from build123d import *

# Parameters (mm, degrees)
F0_W     = 50
F0_H     = 100
F1_DEPTH = 1000
F2_R     = 5.5
F3_T     = -2.5


with BuildPart() as f1:
    # F0 (on Front) → F1 (new body)
    with BuildSketch(Plane.XZ):
        Rectangle(F0_W, F0_H)
    extrude(amount=F1_DEPTH)

    # F2
    f2_edges = [f1.edges().sort_by_distance(p)[0] for p in [
        (-25, -500, 50),
        (25, -500, 50),
        (25, -500, -50),
        (-25, -500, -50),
    ]]
    fillet(f2_edges, radius=F2_R)

    # F3
    f3_openings = [f1.faces().sort_by_distance(p)[0] for p in [
        (0, -1000, 0),
        (0, 0, 0),
    ]]
    offset(amount=F3_T, openings=f3_openings)


solid = f1.part
The listing builds one solid part. Answer for the finished solid, in the listing's coordinates (mm). A direction names the side the tool comes from. Round coordinates to 2 decimals unless told otherwise and drop trailing zeros. Write each loop counter-clockwise with the first axis right and the second up, starting at its lowest first coordinate (ties: lowest second). Pieces come first, ordered by that corner, then holes. Notation, with made-up numbers: (13.25, 76) - (24.25, 76) arc R27 ccw to (24.25, 99) - close; hole circle Ø7 at (0, 63.25). An arc over 180 degrees is marked (long way). Use a Markdown table: item, result. Add a question column.
1. A tool of negligible diameter and unlimited length cuts with its end or side. For faces 1 (the face through (25, -493, -1)), 2 (the face through (22.5, -493, -1)), from which of +Z, -Z, +X, -X, +Y, -Y can it reach the whole face along a straight path? Write none if from no direction.
2. The part is cut by section B-B (y = -574). Write down the section's boundary in (x, z).
3. The part is cut by section A-A (z = -33). Write down the section's boundary in (x, y), and give its area (3 significant figures).
4. For a pull along Z with two mould halves and no side action, classify faces 3 (the face through (0, -493, -47.5)), 4 (the face through (0, -493, 50)), 5 (the face through (-25, -493, -1)), 6 (the face through (-22.5, -493, -1)) as +Z half, -Z half, draft (parallel to the pull), parting line (faces both ways), or undercut.
5. Consider line 1 (Z direction, x = 6, y = -515.5); line 2 (X direction, y = -217.5, z = -28.5); line 3 (Z direction, x = 22, y = -449.5). Determine where each line is inside the solid, lowest interval first.
6. The part is cut by section C-C (x = 3). Write down the section's boundary in (y, z).
Reported:
| question | item | result |
|---|---|---|
| 1 | face 1 | +Z, -Z, +X, +Y, -Y |
| 1 | face 2 | +Y, -Y |
| 2 | outline | (-25, -44.5) arc R5.5 ccw to (-19.5, -50) - (19.5, -50) arc R5.5 ccw to (25, -44.5) - (25, 44.5) arc R5.5 ccw to (19.5, 50) - (-19.5, 50) arc R5.5 ccw to (-25, 44.5) - close; hole (-22.5, -44.5) arc R3 ccw to (-19.5, -47.5) - (19.5, -47.5) arc R3 ccw to (22.5, -44.5) - (22.5, 44.5) arc R3 ccw to (19.5, 47.5) - (-19.5, 47.5) arc R3 ccw to (-22.5, 44.5) - close |
| 3 | outline | (-25, -1000) - (-22.5, -1000) - (-22.5, 0) - (-25, 0) - close; (22.5, -1000) - (25, -1000) - (25, 0) - (22.5, 0) - close |
| 3 | area | 5,000 mm^2 |
| 4 | face 3 | undercut |
| 4 | face 4 | +Z half |
| 4 | face 5 | draft |
| 4 | face 6 | undercut |
| 5 | line 1 | -50 to -47.5, 47.5 to 50 |
| 5 | line 2 | -25 to -22.5, 22.5 to 25 |
| 5 | line 3 | -49.4 to -46.16, 46.16 to 49.4 |
| 6 | outline | (-1000, -50) - (0, -50) - (0, -47.5) - (-1000, -47.5) - close; (-1000, 47.5) - (0, 47.5) - (0, 50) - (-1000, 50) - close |
